Input: part model. Units: mm. Frame: model coordinates. Face numbers are marked on the shaded views. Give positions to 0.01 mm unless a question says otherwise; leave off trailing zeros. Order: outer loops, then holes, each group sorted by start corner. A loop starts at its lowest first (then second) coordinate and runs counter-clockwise, first axis right, second up. Notation, with made-up numbers: (89.5, 40) - (117.5, 40) arc R26 cw to (117.5, 56) - close; hole circle Ø6 at (0, -29). An arc over 180 degrees is marked (long way). Use a Markdown table: item, result.
from build123d import *

# Parameters (mm, degrees)
SKETCH2_W = 0.699473795
SKETCH2_H = 3.65
FILLET1_R = 0.5


with BuildPart() as part:
    # Sketch1 → mainBody (revolve)
    with BuildSketch(Plane(origin=(0, 0, 0), x_dir=(1, 0, 0), z_dir=(0, 1, 0))):
        with BuildLine():
            Line((-30.015877082, 9.1), (30.015877082, 9.1))
            ThreePointArc((30.015877082, 9.1), (30.984122918, 8.85), (31.952368755, 9.1))
            Line((31.952368755, 9.1), (32.984122918, 9.1))
            ThreePointArc((32.984122918, 9.1), (33.691229699, 8.807106781), (33.984122918, 8.1))
            Line((33.984122918, 8.1), (33.984122918, 5.5))
            Line((33.984122918, 5.5), (33.484649123, 5.5))
            Line((33.484649123, 5.5), (33.484649123, 0))
            Line((33.484649123, 0), (-30.715877082, 0))
            Line((-30.715877082, 0), (-30.715877082, 5.5))
            Line((-30.715877082, 5.5), (-31.015877082, 5.5))
            Line((-31.015877082, 5.5), (-31.015877082, 8.1))
            ThreePointArc((-31.015877082, 8.1), (-30.722983863, 8.807106781), (-30.015877082, 9.1))
        make_face()
    revolve(axis=Axis((0, 0, 0), (1, 0, 0)))

    # Sketch2 → Revolve2 (revolve)
    with BuildSketch(Plane(origin=(0, 0, 0), x_dir=(1, 0, 0), z_dir=(0, 1, 0))):
        with Locations((33.834386021, 1.825)):
            Rectangle(SKETCH2_W, SKETCH2_H)
    revolve(axis=Axis((33.484649123, 0, 0), (1, 0, 0)))

    # Fillet1
    fillet1_edges = [part.edges().sort_by_distance(p)[0] for p in [
        (34.184122918, 0, 3.65),
    ]]
    fillet(fillet1_edges, radius=FILLET1_R)


solid = part.part
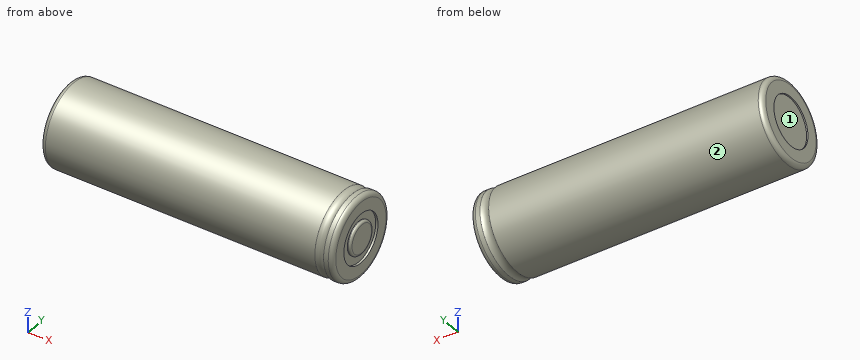
1. Mould query, pull axis Z, two halves, no side actions, for the marked faces 1 and 2. Classes: pulls with the +Z half, pulls with the -Z half, needs draft (parallel to the pull), parting line crosses it, or undercut.
Response:
| item | result |
|---|---|
| face 1 | undercut |
| face 2 | parting line crosses it |
2. Pin query (flat end, axial travel): pin 1 (3.5 mm diameter, centred on y = -2, z = -1, fed in from -X); pin 2 (3 mm diameter, centred on x = -1.5, z = 3.5, fed in from -Y); pin 3 (1 mm diameter, centred on y = -5, z = 5, fed in from +X). Return the tip coordinate at first contact, or that it passes through.
Response:
| item | result |
|---|---|
| pin 1 | stops at x = -30.72 |
| pin 2 | stops at y = -8.88 |
| pin 3 | stops at x = 33.98 |
3. Material intervals for line 1 along Y through (x, z) = (33.7, 0); line 2 along X through (y, z) = (-0.75, -5.5); line 3 along Y through (x, z) = (-30.75, 0), sorted ascending.
Response:
| item | result |
|---|---|
| line 1 | y = -8.8 to -5.5, -3.65 to 3.65, 5.5 to 8.8 |
| line 2 | x = -31.02 to 33.98 |
| line 3 | y = -8.78 to -5.5, 5.5 to 8.78 |
4. Section query A-A (x = 7). Return loops of the section in (y, z), then the cut area to 3 significant figures.
Response:
| item | result |
|---|---|
| outline | circle Ø18.2 at (0, 0) |
| area | 260 mm^2 |
